For this review, take the finished solid that the model builds, in its own axes (mm). A direction names the side the tool comes from. Give positions to 0.01 mm unless a question says otherwise; leave off trailing zeros. Write each loop counter-clockwise with the first axis right and the second up, starting at its lowest first coordinate (ties: lowest second). Pieces come first, ordered by that corner, then holes.
from build123d import *

# Parameters (mm, degrees)
CUT_EXTRUDE1_DEPTH      = 36.212453408
CUT_EXTRUDE1_DEPTH_BACK = 36.212453408
SKETCH3_R               = 2.1828125


with BuildPart() as part:
    # Sketch1 → Revolve2 (revolve)
    with BuildSketch(Plane.XY, mode=Mode.PRIVATE) as revolve2_sk:
        with BuildLine():
            Line((0, 0), (0, 15.875))
            Line((0, 15.875), (15.875, 15.875))
            Line((15.875, 15.875), (15.875, 3.175))
            Line((15.875, 3.175), (22.225, 3.175))
            Line((22.225, 3.175), (22.225, 1.5875))
            ThreePointArc((22.225, 1.5875), (21.760032015, 0.464967985), (20.6375, 0))
            Line((20.6375, 0), (0, 0))
        make_face()
    revolve(revolve2_sk.sketch.rotate(Axis((0, 0, 0), (0, 1, 0)), 90), axis=Axis((0, 0, 0), (0, 1, 0)))

    # Sketch3 → Cut-Extrude1 (cut, two sides: drawn at the far end of the back side and taken through both)
    with BuildSketch(Plane(origin=(0, 15.875, 0), x_dir=(1, 0, 0), z_dir=(0, 1, 0)).offset(-CUT_EXTRUDE1_DEPTH_BACK)):
        with Locations(Location((0, 0, 0), (0, 0, 270))):
            Circle(SKETCH3_R)
        with Locations(Location((12.7, 0, 0), (0, 0, 270))):
            Circle(SKETCH3_R)
        with Locations(Location((-12.7, 0, 0), (0, 0, 270))):
            Circle(SKETCH3_R)
        with Locations(Location((0, -12.7, 0), (0, 0, 270))):
            Circle(SKETCH3_R)
        with Locations(Location((0, 12.7, 0), (0, 0, 270))):
            Circle(SKETCH3_R)
    extrude(amount=CUT_EXTRUDE1_DEPTH + CUT_EXTRUDE1_DEPTH_BACK, mode=Mode.SUBTRACT)


solid = part.part
(1) Tool access review of faces 5 (the flat face through (0, 15.875, 3)), 6 (the flat face through (15, 3.175, 10)): name each direction out of +Z, -Z, +X, -X, +Y, -Y from which nothing blocks a thin tool from reaching the whole face with its end or side.
(2) The part is to be moulded in two halves that separate along X. For faces 1 (the cylindrical face through (-15, 2.4, 16.4)), 2 (the flat face through (4, 0, 0)), 3 (the cylindrical face through (-1.33, 7.83, 10.97)), 4 (the cylindrical face through (-2.13, 7.83, -0.47)), say which applies: +X half, -X half, draft (parallel to the pull), parting line (faces both ways), or undercut.
(3) We need section A-A (x = 0). Write out the cut boundary in (y, z) (1 decimal), and give its area (3 significant figures).
(4) We need section B-B (z = 0). Write out the cut boundary in (x, y) (1 decimal), and give its area (3 significant figures).
(5) For L1, parallel to X at y = 4.5, z = 0 (3 decimals); L2, parallel to X at y = 11.5, z = 1; L3, parallel to Z at x = -0.5, y = 8.5, list the stretches that pass through material, from the lowest coordinate up.
(6) We need section C-C (y = 6). Write out the cut boundary in (x, z) (3 decimals).
(7) Clearance check with flat-ended pins moving along their axes: pin 1 Ø2 at (y, z) = (8, -3) entering from +X; pin 2 Ø3 at (y, z) = (11.5, 5.5) entering from +X; pin 3 Ø8 at (y, z) = (4.5, -0.5) entering from +X (3 decimals). State where each tip first meets the part, or that it passes through.
The answers:
1. face 5: +Z, -Z, +X, -X, +Y
1. face 6: +Y
2. face 1: parting line
2. face 2: draft
2. face 3: undercut
2. face 4: undercut
3. outline: (0, -20.6) arc R1.6 ccw to (1.6, -22.2) - (3.2, -22.2) - (3.2, -15.9) - (15.9, -15.9) - (15.9, -14.9) - (0, -14.9) - close; (0, -10.5) - (15.9, -10.5) - (15.9, -2.2) - (0, -2.2) - close; (0, 2.2) - (15.9, 2.2) - (15.9, 10.5) - (0, 10.5) - close; (0, 14.9) - (15.9, 14.9) - (15.9, 15.9) - (3.2, 15.9) - (3.2, 22.2) - (1.6, 22.2) arc R1.6 ccw to (0, 20.6) - close
3. area: 335 mm2
4. outline: (-22.2, 1.6) arc R1.6 ccw to (-20.6, 0) - (-14.9, 0) - (-14.9, 15.9) - (-15.9, 15.9) - (-15.9, 3.2) - (-22.2, 3.2) - close; (-10.5, 0) - (-2.2, 0) - (-2.2, 15.9) - (-10.5, 15.9) - close; (2.2, 0) - (10.5, 0) - (10.5, 15.9) - (2.2, 15.9) - close; (14.9, 0) - (20.6, 0) arc R1.6 ccw to (22.2, 1.6) - (22.2, 3.2) - (15.9, 3.2) - (15.9, 15.9) - (14.9, 15.9) - close
4. area: 335 mm2
5. L1: x = -15.875 to -14.883, -10.517 to -2.183, 2.183 to 10.517, 14.883 to 15.875
5. L2: x = -15.84 to -14.64, -10.76 to -1.94, 1.94 to 10.76, 14.64 to 15.84
5. L3: z = -15.87 to -14.82, -10.58 to -2.12, 2.12 to 10.58, 14.82 to 15.87
6. outline: circle Ø31.75 at (0, 0); hole circle Ø4.366 at (-12.7, 0); hole circle Ø4.366 at (0, -12.7); hole circle Ø4.366 at (0, 0); hole circle Ø4.366 at (0, 12.7); hole circle Ø4.366 at (12.7, 0)
7. pin 1: stops at x = 15.75
7. pin 2: stops at x = 15.36
7. pin 3: stops at x = 22.225
